Here's the drawing with two shaded views (mm, measured from the low corner). I have some questions. A direction names the side the tool comes from. Coordinates: 2 decimals unless noted, no trailing zeros. Order: outer loops, then holes, each group sorted by start corner. A loop starts at its lowest first (then second) coordinate and runs counter-clockwise, first axis right, second up. Notation, with made-up numbers: (-20.75, 37.5) -> (7.25, 37.5) arc R35 cw to (7.25, 72.5) -> close; hole circle Ø11 at (45.25, -18). An arc over 180 degrees is marked (long way). One line per item, written item: value. Start each with the question number.
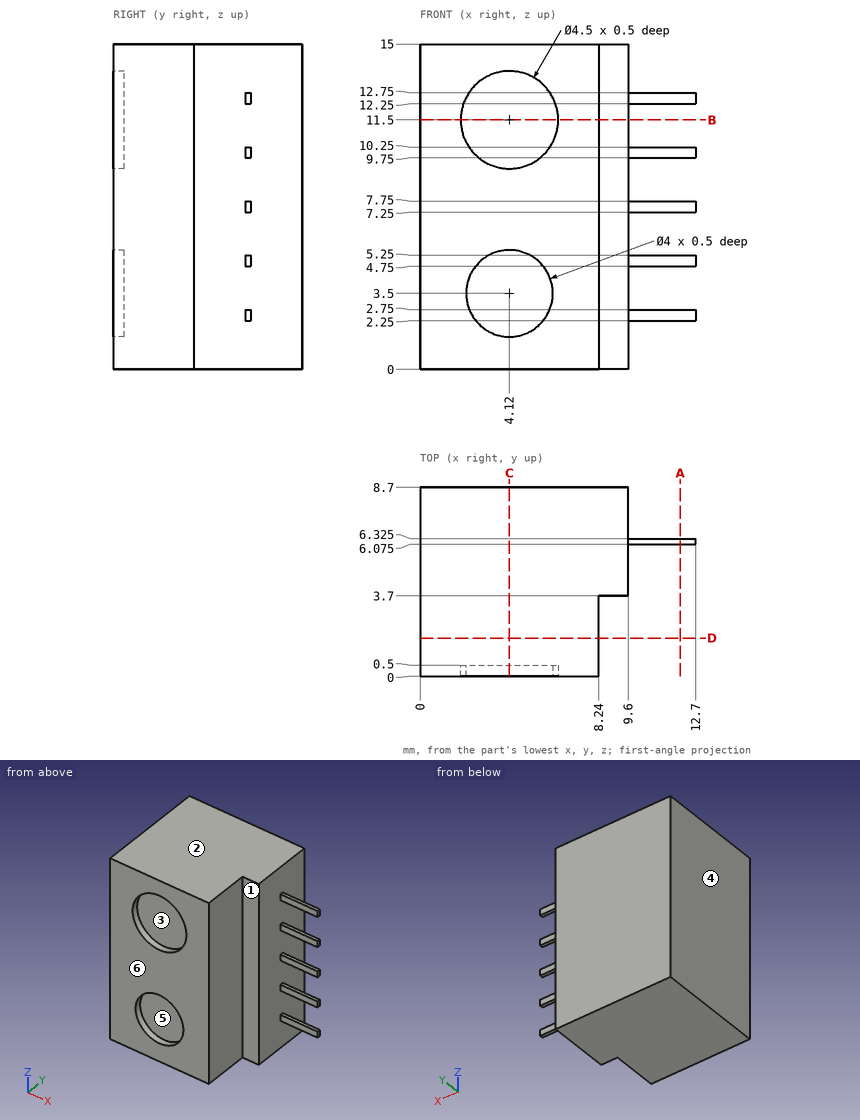
Q1. I need wall thicknesses on line 1 (Z direction, x = 4.12, y = 0.4); line 2 (X direction, y = 0.15, z = 11.5); line 3 (X direction, y = 3.5, z = 12.75). Which ranges of each line are inside material? Lowest first, please.
Q2. Imagine slicing it at B-B (z = 11.5). Write out the boundary of the cut face in (x, y).
Q3. For P1, Ø5, axis at y = 2.5, z = 3.5, coming from the +X side; P2, Ø1, axis at x = 9.5, y = 2, coming from the -Z side; P3, Ø2, axis at x = 4, z = 11.5, coming from the -Y side, each with a flat end and sliding along its axis, tell me the tip position at first contact or that it passes through.
Q4. Imagine slicing it at D-D (y = 1.75). Write out the boundary of the cut face in (x, z).
Q5. Imagine slicing it at C-C (x = 4.12). Write out the boundary of the cut face in (y, z), plus the area to 3 significant figures.
Q6. Imagine slicing it at A-A (x = 12). Write out the boundary of the cut face in (y, z) (3 decimals).
Q7. For the marked faces 1 and 2, which set-ups out of +Z, -Z, +X, -X, +Y, -Y let a thin tool reach every point of the face, with its end or its side?
Q8. If we mould it in two halves opening along X, with no side actions, what happens to the marked faces 3, 4, 5 and 6? For each: +X half, -X half, draft (parallel to the pull), parting line (faces both ways), or undercut.
Completed:
1. line 1: z = 0 to 1.5, 5.5 to 9.25, 13.75 to 15
1. line 2: x = 0 to 1.87, 6.37 to 8.24
1. line 3: x = 0 to 8.24
2. outline: (0, 0) -> (1.87, 0) -> (1.87, 0.5) -> (6.37, 0.5) -> (6.37, 0) -> (8.24, 0) -> (8.24, 3.7) -> (9.6, 3.7) -> (9.6, 8.7) -> (0, 8.7) -> close
3. P1: stops at x = 9.6
3. P2: passes through
3. P3: stops at y = 0.5
4. outline: (0, 0) -> (8.24, 0) -> (8.24, 15) -> (0, 15) -> close
5. outline: (0, 0) -> (8.7, 0) -> (8.7, 15) -> (0, 15) -> (0, 13.75) -> (0.5, 13.75) -> (0.5, 9.25) -> (0, 9.25) -> (0, 5.5) -> (0.5, 5.5) -> (0.5, 1.5) -> (0, 1.5) -> close
5. area: 126 mm2
6. outline: (6.075, 2.25) -> (6.325, 2.25) -> (6.325, 2.75) -> (6.075, 2.75) -> close; (6.075, 4.75) -> (6.325, 4.75) -> (6.325, 5.25) -> (6.075, 5.25) -> close; (6.075, 7.25) -> (6.325, 7.25) -> (6.325, 7.75) -> (6.075, 7.75) -> close; (6.075, 9.75) -> (6.325, 9.75) -> (6.325, 10.25) -> (6.075, 10.25) -> close; (6.075, 12.25) -> (6.325, 12.25) -> (6.325, 12.75) -> (6.075, 12.75) -> close
7. face 1: +Z, -Z, +X, -Y
7. face 2: +Z, +X, -X, +Y, -Y
8. face 3: undercut
8. face 4: -X half
8. face 5: undercut
8. face 6: draft
